```python
from build123d import *

# Parameters (mm, degrees)
SKETCH_1_R      = 1.5
EXTRUDE_1_DEPTH = 2


with BuildPart() as part:
    # 草图1 → 凸台-拉伸1 (new body)
    with BuildSketch(Plane.XY):
        with BuildLine():
            Line((-8.682938962, -11.200971973), (-10.682938962, -11.200971973))
            Line((-10.682938962, -11.200971973), (-10.682938962, -6.200971973))
            Line((-10.682938962, -6.200971973), (-8.682938962, -6.200971973))
            Line((-8.682938962, -6.200971973), (-8.682938962, -2.700971973))
            Line((-8.682938962, -2.700971973), (-6.182938962, -2.700971973))
            Line((-6.182938962, -2.700971973), (-6.182938962, -4.200971973))
            Line((-6.182938962, -4.200971973), (-3.582938962, -4.200971973))
            Line((-3.582938962, -4.200971973), (-3.582938962, -2.700971973))
            Line((-3.582938962, -2.700971973), (-0.582938962, -2.700971973))
            Line((-0.582938962, -2.700971973), (-0.582938962, 0.299028027))
            Line((-0.582938962, 0.299028027), (-3.582938962, 0.299028027))
            Line((-3.582938962, 0.299028027), (-3.582938962, 1.799028027))
            Line((-3.582938962, 1.799028027), (-6.182938962, 1.799028027))
            Line((-6.182938962, 1.799028027), (-6.182938962, 0.299028027))
            Line((-6.182938962, 0.299028027), (-8.682938962, 0.299028027))
            Line((-8.682938962, 0.299028027), (-8.682938962, 3.799028027))
            Line((-8.682938962, 3.799028027), (-10.682938962, 3.799028027))
            Line((-10.682938962, 3.799028027), (-10.682938962, 8.799028027))
            Line((-10.682938962, 8.799028027), (-8.682938962, 8.799028027))
            Line((-8.682938962, 8.799028027), (-8.682938962, 10.799028027))
            Line((-8.682938962, 10.799028027), (-3.582938962, 10.799028027))
            ThreePointArc((-3.582938962, 10.799028027), (-2.532938962, 9.749028027), (-1.482938962, 10.799028027))
            Line((-1.482938962, 10.799028027), (16.317061038, 10.799028027))
            Line((16.317061038, 10.799028027), (16.317061038, 8.799028027))
            Line((16.317061038, 8.799028027), (18.317061038, 8.799028027))
            Line((18.317061038, 8.799028027), (18.317061038, 3.799028027))
            Line((18.317061038, 3.799028027), (16.317061038, 3.799028027))
            Line((16.317061038, 3.799028027), (16.317061038, 0.299028027))
            Line((16.317061038, 0.299028027), (13.817061038, 0.299028027))
            Line((13.817061038, 0.299028027), (13.817061038, 1.799028027))
            Line((13.817061038, 1.799028027), (11.217061038, 1.799028027))
            Line((11.217061038, 1.799028027), (11.217061038, 0.299028027))
            Line((11.217061038, 0.299028027), (8.217061038, 0.299028027))
            Line((8.217061038, 0.299028027), (8.217061038, -2.700971973))
            Line((8.217061038, -2.700971973), (11.217061038, -2.700971973))
            Line((11.217061038, -2.700971973), (11.217061038, -4.200971973))
            Line((11.217061038, -4.200971973), (13.817061038, -4.200971973))
            Line((13.817061038, -4.200971973), (13.817061038, -2.700971973))
            Line((13.817061038, -2.700971973), (16.317061038, -2.700971973))
            Line((16.317061038, -2.700971973), (16.317061038, -6.200971973))
            Line((16.317061038, -6.200971973), (18.317061038, -6.200971973))
            Line((18.317061038, -6.200971973), (18.317061038, -11.200971973))
            Line((18.317061038, -11.200971973), (16.317061038, -11.200971973))
            Line((16.317061038, -11.200971973), (16.317061038, -15.200971973))
            Line((16.317061038, -15.200971973), (4.222987954, -15.200971973))
            Line((4.222987954, -15.200971973), (3.817061038, -15.955763704))
            Line((3.817061038, -15.955763704), (3.411134121, -15.200971973))
            Line((3.411134121, -15.200971973), (-8.682938962, -15.200971973))
            Line((-8.682938962, -15.200971973), (-8.682938962, -11.200971973))
        make_face()
        with Locations((3.817061038, -6.200971973)):
            Circle(SKETCH_1_R, mode=Mode.SUBTRACT)
        with Locations((3.817061038, 3.799028027)):
            Circle(SKETCH_1_R, mode=Mode.SUBTRACT)
        with Locations((3.817061038, -12.192801434)):
            Circle(SKETCH_1_R, mode=Mode.SUBTRACT)
        with BuildLine():
            Line((13.267061038, -13.342801434), (7.967061038, -13.342801434))
            ThreePointArc((7.967061038, -13.342801434), (7.490715441, -12.192801434), (7.967061038, -11.042801434))
            Line((7.967061038, -11.042801434), (13.267061038, -11.042801434))
            Line((13.267061038, -11.042801434), (13.267061038, -13.342801434))
        make_face(mode=Mode.SUBTRACT)
        with BuildLine():
            Line((-5.632938962, -11.042801434), (-0.332938962, -11.042801434))
            ThreePointArc((-0.332938962, -11.042801434), (0.143406634, -12.192801434), (-0.332938962, -13.342801434))
            Line((-0.332938962, -13.342801434), (-5.632938962, -13.342801434))
            Line((-5.632938962, -13.342801434), (-5.632938962, -11.042801434))
        make_face(mode=Mode.SUBTRACT)
    extrude(amount=EXTRUDE_1_DEPTH)


solid = part.part
```
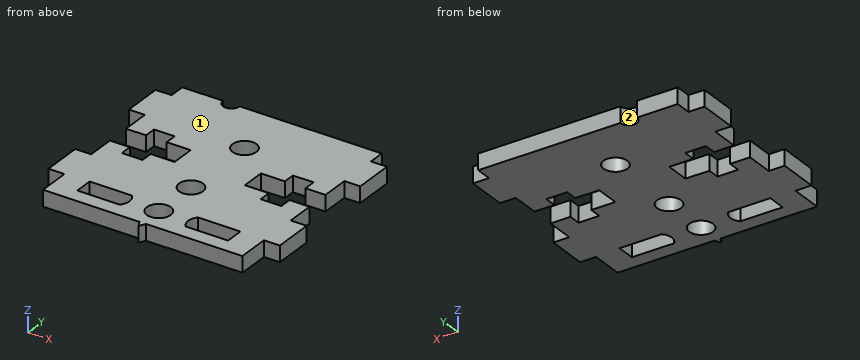
Design review of the part built by this model. Coordinates are the model's own, in mm. Face numbers are marked on the shaded views. Round coordinates to 2 decimals unless told otherwise and drop trailing zeros. Write each loop counter-clockwise with the first axis right and the second up, starting at its lowest first coordinate (ties: lowest second). Pieces come first, ordered by that corner, then holes. Notation, with made-up numbers: (28.25, -2.5) -> (71.25, -2.5) arc R20 cw to (71.25, 19.5) -> close; hole circle Ø6 at (12.5, -4). An arc over 180 degrees is marked (long way). Answer in a Markdown table with one row per item.
Q1. Take a section at C-C, the plane x = 0.75. State the section outline as (y, z) points, then the cut area to 3 significant figures.
The answers:
| item | result |
|---|---|
| outline | (-15.2, 0) -> (10.8, 0) -> (10.8, 2) -> (-15.2, 2) -> close |
| area | 52.0 mm² |
Q2. Take a section at B-B, the plane z = 1.65. Count the separate pieces of the cut face and the enclosed holes in it, then the cut area to 3 significant figures.
The answers:
| item | result |
|---|---|
| separate pieces | 1 |
| enclosed holes | 5 |
| area | 577 mm² |
Q3. Clearance check with flat-ended pins moving along their axes: pin 1 Ø0.8 at (y, z) = (1, 1) entering from -X; pin 2 Ø0.6 at (y, z) = (-1.5, 0.5) entering from -X; pin 3 Ø1 at (x, z) = (12.5, 1) entering from -Y. State where each tip first meets the part, or that it passes through.
The answers:
| item | result |
|---|---|
| pin 1 | x = -8.68 |
| pin 2 | x = -0.58 |
| pin 3 | y = -15.2 |
Q4. To check wall thickness, follow L1, parallel to X at y = 1.5, z = 1.15; L2, parallel to Y at x = 10.5, z = 1.7; L3, parallel to Y at x = 11.75, z = 1.95. State the ranges of each line that lie inside material, in increasing order. Write a range as [from, to].
The answers:
| item | result |
|---|---|
| L1 | [-8.68, -6.18], [-3.58, 11.22], [13.82, 16.32] |
| L2 | [-15.2, -13.34], [-11.04, -2.7], [0.3, 10.8] |
| L3 | [-15.2, -13.34], [-11.04, -4.2], [1.8, 10.8] |
Q5. Take a section at A-A, the plane y = -5.5. State the section outline as (x, z) points.
The answers:
| item | result |
|---|---|
| outline | (-8.68, 0) -> (2.49, 0) -> (2.49, 2) -> (-8.68, 2) -> close; (5.14, 0) -> (16.32, 0) -> (16.32, 2) -> (5.14, 2) -> close |
Q6. Take a section at D-D, the plane y = -1.25. State the section outline as (x, z) points.
The answers:
| item | result |
|---|---|
| outline | (-0.58, 0) -> (8.22, 0) -> (8.22, 2) -> (-0.58, 2) -> close |
Q7. Draft analysis for pull direction X (two halves, no side actions). For the marked faces 1 and 2, state which applies: +X half, -X half, draft (parallel to the pull), parting line (faces both ways), or undercut.
The answers:
| item | result |
|---|---|
| face 1 | draft |
| face 2 | undercut |
